Part model, mm, in its own coordinate system. A direction names the side the tool comes from. Give positions to 0.01 mm unless a question says otherwise; leave off trailing zeros. Write each loop counter-clockwise with the first axis right and the second up, starting at its lowest first coordinate (ties: lowest second). Pieces come first, ordered by that corner, then holes. Notation, with made-up numbers: M -3.5,77.25 L 46.5,77.25 A21 cw 46.5,109.25 Z; hole C -31,-37 d2. An arc over 180 degrees is marked long. Use a Markdown table: item, result.
```python
from build123d import *

# Parameters (mm, degrees)
SKETCH2_R          = 2
CUT_EXTRUDE1_DEPTH = 21
SKETCH3_R          = 3.25
CUT_EXTRUDE2_DEPTH = 21
CIRPATTERN1_COUNT  = 4
CIRPATTERN2_COUNT  = 3


with BuildPart() as part:
    # Sketch1 → Revolve1 (revolve)
    with BuildSketch(Plane.XY):
        Polygon((13, 0), (13, 5), (25, 5), (25, 20), (40, 20), (40, 0), align=None)
    revolve(axis=Axis((0, 51.395093442, 0), (0, -1, 0)))

    # Sketch2 → Cut-Extrude1 (cut, through all)
    with BuildSketch(Plane(origin=(0, 20, 0), x_dir=(1, 0, 0), z_dir=(0, 1, 0))):
        with Locations((-17.5, 0)):
            Circle(SKETCH2_R)
    cut_extrude1 = extrude(amount=-CUT_EXTRUDE1_DEPTH, mode=Mode.SUBTRACT)

    # Sketch3 → Cut-Extrude2 (cut, through all)
    with BuildSketch(Plane(origin=(0, 20, 0), x_dir=(1, 0, 0), z_dir=(0, 1, 0))):
        with Locations((0, 32)):
            Circle(SKETCH3_R)
    cut_extrude2 = extrude(amount=-CUT_EXTRUDE2_DEPTH, mode=Mode.SUBTRACT)

    # CirPattern1: Cut-Extrude2 ×4 about axis
    cirpattern1_axis = Axis((0, 0, 0), (0, 1, 0))
    for i in range(1, CIRPATTERN1_COUNT):
        add(cut_extrude2.rotate(cirpattern1_axis, i * 360 / CIRPATTERN1_COUNT), mode=Mode.SUBTRACT)

    # CirPattern2: Cut-Extrude1 ×3 about axis
    cirpattern2_axis = Axis((0, 0, 0), (0, 1, 0))
    for i in range(1, CIRPATTERN2_COUNT):
        add(cut_extrude1.rotate(cirpattern2_axis, i * 360 / CIRPATTERN2_COUNT), mode=Mode.SUBTRACT)


solid = part.part
```
1. Tool access for faces 4 (the cylindrical face through (23.846, 12.605, 7.509)), 5 (the cylindrical face through (-28.827, 10.14, 0.705)): list every direction of +Z, -Z, +X, -X, +Y, -Y with a clear straight run to the whole face (end or side of a thin tool).
Findings below:
| item | result |
|---|---|
| face 4 | +Y |
| face 5 | +Y, -Y |
2. Cut at B-B, the plane x = 32. Give the cut face in (y, z).
Findings below:
| item | result |
|---|---|
| outline | M 0,-24 L 20,-24 L 20,-3.25 L 0,-3.25 Z; M 0,3.25 L 20,3.25 L 20,24 L 0,24 Z |
3. Cut at C-C, the plane y = 7.75. Give the cut face in (x, z), then the cut area to 3 significant figures.
Findings below:
| item | result |
|---|---|
| outline | C 0,0 d80; hole C -32,0 d6.5; hole C 0,0 d50; hole C 0,-32 d6.5; hole C 0,32 d6.5; hole C 32,0 d6.5 |
| area | 2,930 mm2 |
4. Cut at D-D, the plane x = 8.75. Give the cut face in (y, z), then the cut area to 3 significant figures.
Findings below:
| item | result |
|---|---|
| outline | M 0,-39.03 L 20,-39.03 L 20,-23.42 L 5,-23.42 L 5,-17.16 L 0,-17.16 Z; M 0,-13.16 L 5,-13.16 L 5,-9.61 L 0,-9.61 Z; M 0,9.61 L 5,9.61 L 5,13.16 L 0,13.16 Z; M 0,17.16 L 5,17.16 L 5,23.42 L 20,23.42 L 20,39.03 L 0,39.03 Z |
| area | 723 mm2 |
5. Drop flat-ended pins along their axis: P1, Ø1, axis at x = 23, z = 3.5, coming from the +Y side; P2, Ø1.5, axis at x = 22.5, y = 10, coming from the -Z side; P3, Ø10, axis at y = 9, z = -28.5, coming from the +X side; P4, Ø8.5, axis at x = 32, z = 0, coming from the +Y side. Give the stop position or say it passes through.
Findings below:
| item | result |
|---|---|
| P1 | y = 5 |
| P2 | z = -33.57 |
| P3 | x = 32.37 |
| P4 | y = 20 |
6. Two-plate mould, pull along X, no slides. Class faces 1 (the cylindrical face through (-8.67, 9.86, -39.05)), 2 (the flat face through (-17.22, 20, 18.34)), 3 (the cylindrical face through (7.16, 2.54, 16.37)): released by +X, released by -X, zero draft, split by the parting line, or undercut.
Findings below:
| item | result |
|---|---|
| face 1 | split by the parting line |
| face 2 | zero draft |
| face 3 | undercut |
7. Drill centre lines: L1, parallel to Z at x = 0, y = 10.5; L2, parallel to X at y = 9.75, z = 1.5; L3, parallel to Z at x = 8, y = 1.75. Where is each one in solid material? Low to high.
Findings below:
| item | result |
|---|---|
| L1 | -40 to -35.25, -28.75 to -25, 25 to 28.75, 35.25 to 40 |
| L2 | -39.97 to -34.88, -29.12 to -24.95, 24.95 to 29.12, 34.88 to 39.97 |
| L3 | -39.19 to -17.01, -13.3 to -10.25, 10.25 to 13.3, 17.01 to 39.19 |
8. Cut at A-A, the plane z = -32. Give the cut face in (x, y), then the cut area to 3 significant figures.
Findings below:
| item | result |
|---|---|
| outline | M -24,0 L -3.25,0 L -3.25,20 L -24,20 Z; M 3.25,0 L 24,0 L 24,20 L 3.25,20 Z |
| area | 830 mm2 |
